Here's how the part is built. I have some questions about the finished solid (model axes, mm). A direction names the side the tool comes from. Coordinates: 2 decimals unless noted, no trailing zeros. Loops run counter-clockwise (first coordinate to the right, second up) from the corner with the lowest first, then second, coordinate; pieces in that order, holes last.
from build123d import *

# Parameters (mm, degrees)
BOSS_EXTRUDE1_DEPTH = 21
CUT_EXTRUDE1_DEPTH  = 22.662179022
BOSS_EXTRUDE2_DEPTH = 49
FILLET1_R           = 0.4
SKETCH4_W           = 7.390362968
SKETCH4_H           = 6.925637862
CUT_EXTRUDE2_DEPTH  = 4.5


with BuildPart() as part:
    # Sketch1 → Boss-Extrude1 (new body)
    with BuildSketch(Plane.XY):
        Polygon((0, 0), (2, 0), (2, 2), (3.5, 2), (3.5, -4), (2, -4), (2, -2), (0, -2), (0, -4), (-1.5, -4), (-1.5, 2), (0, 2), align=None)
    extrude(amount=BOSS_EXTRUDE1_DEPTH)

    # Sketch2 → Cut-Extrude1 (cut, through all)
    with BuildSketch(Plane.XY.offset(21)):
        Polygon((-1.5, 2), (-1.5, 1.9), (-0.1, 1.9), (-0.1, -0.1), (2.1, -0.1), (2.1, 1.9), (3.5, 1.9), (3.5, 2), align=None)
        Polygon((-1.5, -4), (3.5, -4), (3.5, -3.9), (2.1, -3.9), (2.1, -1.9), (-0.1, -1.9), (-0.1, -3.9), (-1.5, -3.9), align=None)
    extrude(amount=-CUT_EXTRUDE1_DEPTH, mode=Mode.SUBTRACT)

    # Sketch3 → Boss-Extrude2 (add)
    with BuildSketch(Plane(origin=(0, 0, 0), x_dir=(-1, 0, 0), z_dir=(0, 0, -1))):
        Polygon((-2.1, -0.1), (-2.1, 1.9), (-3.5, 1.9), (-3.5, -3.9), (-2.1, -3.9), (-2.1, -1.9), (0.1, -1.9), (0.1, -3.9), (1.5, -3.9), (1.5, 1.9), (0.1, 1.9), (0.1, -0.1), align=None)
    extrude(amount=BOSS_EXTRUDE2_DEPTH)

    # Fillet1
    fillet1_edges = [part.edges().sort_by_distance(p)[0] for p in [
        (3.5, 1.9, -14),
        (2.1, 1.9, -14),
        (-0.1, 1.9, -14),
        (-1.5, 1.9, -14),
        (-1.5, -3.9, -14),
        (-0.1, -3.9, -14),
        (2.1, -3.9, -14),
        (3.5, -3.9, -14),
    ]]
    fillet(fillet1_edges, radius=FILLET1_R)

    # Sketch4 → Cut-Extrude2 (cut)
    with BuildSketch(Plane.XY.offset(21)):
        with Locations((1.359853511, -0.992123471)):
            Rectangle(SKETCH4_W, SKETCH4_H)
    extrude(amount=-CUT_EXTRUDE2_DEPTH, mode=Mode.SUBTRACT)


solid = part.part
Q1. Please list where these lines run through material, in increasing order: probe 1 along X at (y, z) = (-2.8, -3); probe 2 along Y at (x, z) = (1.9, -23); probe 3 along Y at (x, z) = (2.3, -41.5).
Q2. Suppose I cut it at A-A on y = 0.75. Write out the boundary of the cut face in (x, z), and give its area (3 significant figures).
Q3. Suppose I cut it at B-B on z = 6. Write out the boundary of the cut face in (x, y), and give its area (3 significant figures).
Q4. We'd pull the mould along X, two halves only. Please class faces 1 (the flat face through (-1.5, -1, -16)), 2 (the flat face through (-0.1, 1, -16)), 3 (the flat face through (1, -1, -49)), 4 (the flat face through (-0.1, -3, -16)): pulls with the +X half, pulls with the -X half, needs draft (parallel to the pull), parting line crosses it, or undercut.
Q5. Will this pin go through, and if not, where does the flat tip stop? P1, Ø1.1, axis at x = 1, z = -9, coming from the -Y side.
Q6. For faces 5 (the flat face through (1, -1.9, -16)), 6 (the flat face through (3.5, -1, -16)), 7 (the flat face through (1, -0.1, -16)), which set-ups out of +Z, -Z, +X, -X, +Y, -Y let a thin tool reach every point of the face, with its end or its side?
Q7. Suppose I cut it at C-C on x = 1.5. Write out the boundary of the cut face in (y, z), and give its area (3 significant figures).
Check values:
1. probe 1: x = -1.5 to -0.1, 2.1 to 3.5
1. probe 2: y = -1.9 to -0.1
1. probe 3: y = -3.85 to 1.85
2. outline: (-1.5, -49) - (-0.1, -49) - (-0.1, 16.5) - (-1.5, 16.5) - close; (2.1, -49) - (3.5, -49) - (3.5, 16.5) - (2.1, 16.5) - close
2. area: 183 mm2
3. outline: (-1.5, -3.5) arc R0.4 ccw to (-1.1, -3.9) - (-0.5, -3.9) arc R0.4 ccw to (-0.1, -3.5) - (-0.1, -1.9) - (2.1, -1.9) - (2.1, -3.5) arc R0.4 ccw to (2.5, -3.9) - (3.1, -3.9) arc R0.4 ccw to (3.5, -3.5) - (3.5, 1.5) arc R0.4 ccw to (3.1, 1.9) - (2.5, 1.9) arc R0.4 ccw to (2.1, 1.5) - (2.1, -0.1) - (-0.1, -0.1) - (-0.1, 1.5) arc R0.4 ccw to (-0.5, 1.9) - (-1.1, 1.9) arc R0.4 ccw to (-1.5, 1.5) - close
3. area: 19.9 mm2
4. face 1: pulls with the -X half
4. face 2: undercut
4. face 3: needs draft
4. face 4: undercut
5. P1: stops at y = -1.9
6. face 5: +Z, -Z, -Y
6. face 6: +Z, -Z, +X, +Y, -Y
6. face 7: +Z, -Z, +Y
7. outline: (-1.9, -49) - (-0.1, -49) - (-0.1, 16.5) - (-1.9, 16.5) - close
7. area: 118 mm2
